The figure shows three views and two pictorial views of one solid part (mm, origin at its lowest corner). Answer the questions. A direction names the side the tool comes from. Give positions to 0.01 mm unless a question says otherwise; leave off trailing zeros. Write each loop counter-clockwise with the first axis right and the second up, starting at its lowest first coordinate (ties: lowest second). Pieces come first, ordered by that corner, then holes. Notation, with made-up numbers: (48.25, -0.75) -> (55.25, -0.75) arc R28 cw to (55.25, 27.25) -> close; hole circle Ø1 at (63, 73.25). An arc over 180 degrees is marked (long way). Answer as CSV lines item,"result". Start each with the question number.
1. Given pin 1 (10 mm diameter, centred on x = 54.5, y = 55.5, fed in from -Z); pin 2 (6.5 mm diameter, centred on x = 20, y = 21, fed in from +Z); pin 3 (8.5 mm diameter, centred on y = 38, z = 24, fed in from +X); pin 4 (3 mm diameter, centred on y = 12.5, z = 34.5, fed in from +X), each flat-ended and moving along its own axis, determine where each tip first touches the part or whether it passes through.
2. A tool of negligible diameter and unlimited length cuts with its end or side. For the marked faces 4, 5 and 6, from which of +Z, -Z, +X, -X, +Y, -Y can it reach the whole face along a straight path? Write none if from no direction.
3. The part is cut by section A-A, the plane z = 9. Determine the outline of the cut face in (x, y) (1 decimal), and give its area (3 significant figures).
4. The part is cut by section D-D, the plane y = 36. Determine the outline of the cut face in (x, z), and give its area (3 significant figures).
5. The part is cut by section C-C, the plane x = 18. Determine the outline of the cut face in (y, z), and give its area (3 significant figures).
6. For a pull along X with two mould halves and no side action, classify the marked faces 1, 2 and 3 as pulls with the +X half, pulls with the -X half, needs draft (parallel to the pull), parting line crosses it, or undercut.
7. Find the intervals of material crossed by line 1 (X direction, y = 57.5, z = 41.5); line 2 (Z direction, x = 28.5, y = 23); line 3 (Y direction, x = 16, z = 54), in increasing order.
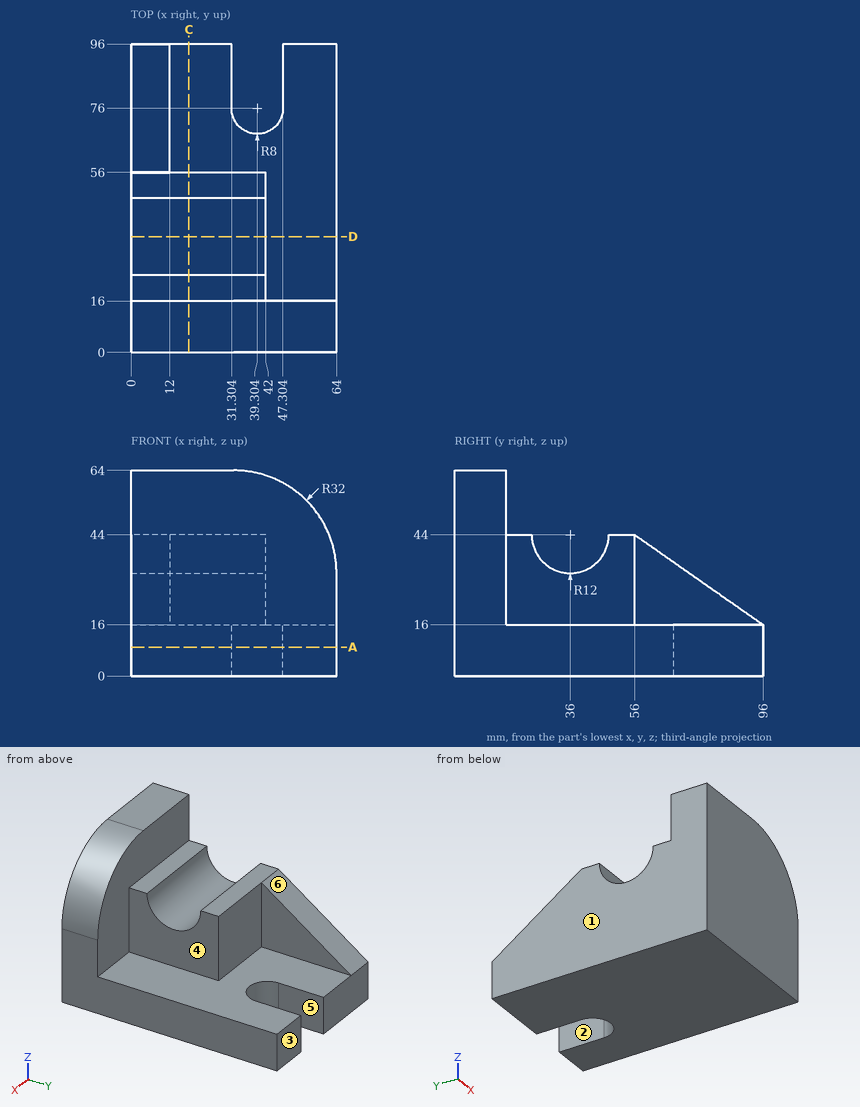
Results found:
1,pin 1,"stops at z = 0"
1,pin 2,"stops at z = 44"
1,pin 3,"stops at x = 42"
1,pin 4,"stops at x = 63.98"
2,face 4,"+Z, +X, +Y"
2,face 5,"+Z, -Z, +Y"
2,face 6,"+Z, +X, -X, +Y"
3,outline,"(0, 0) -> (64, 0) -> (64, 96) -> (47.3, 96) -> (47.3, 76) arc R8 cw to (31.3, 76) -> (31.3, 96) -> (0, 96) -> close"
3,area,"5,720 mm²"
4,outline,"(0, 0) -> (64, 0) -> (64, 16) -> (42, 16) -> (42, 32) -> (0, 32) -> close"
4,area,"1,700 mm²"
5,outline,"(0, 0) -> (96, 0) -> (96, 16) -> (56, 16) -> (56, 44) -> (48, 44) arc R12 cw to (24, 44) -> (16, 44) -> (16, 64) -> (0, 64) -> close"
5,area,"3,200 mm²"
6,face 1,"pulls with the -X half"
6,face 2,"undercut"
6,face 3,"needs draft"
7,line 1,"x = 0 to 12"
7,line 2,"z = 0 to 44"
7,line 3,"y = 0 to 16"
